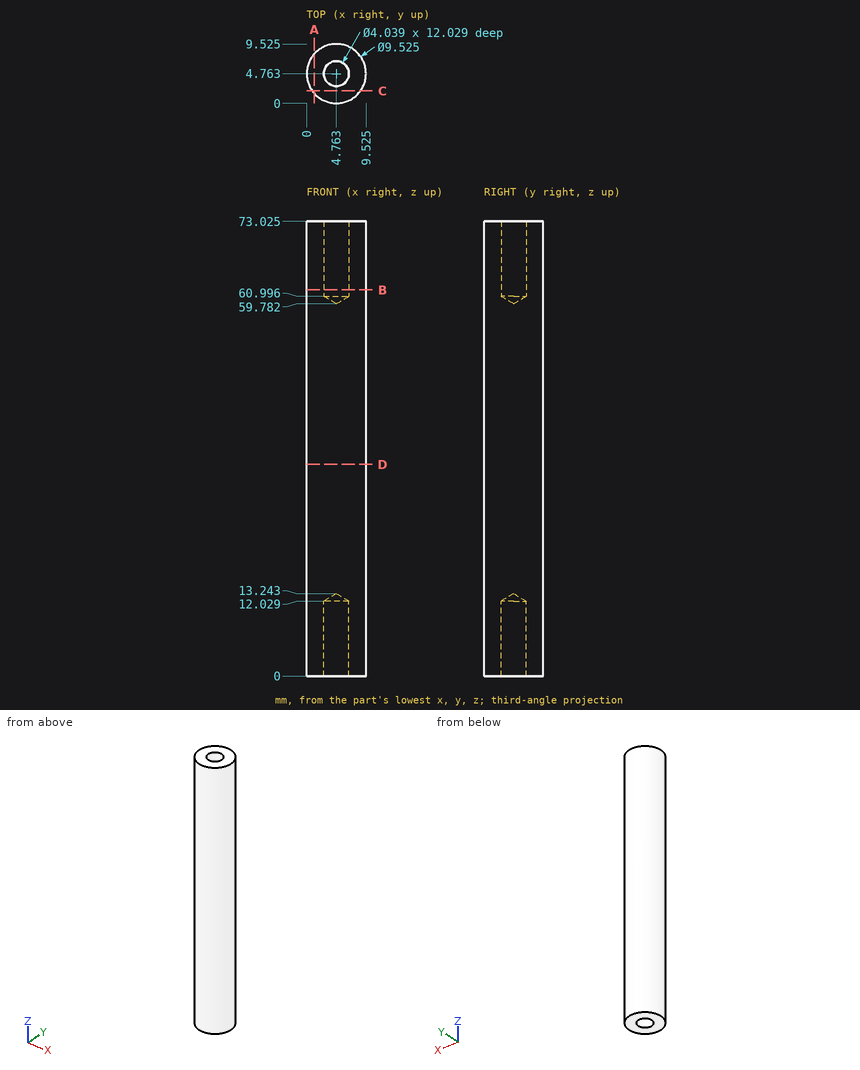
The drawing under review shows one solid part. Ordinate dimensions are in mm from its lowest x, y, z. Round coordinates to 2 decimals unless told otherwise and drop trailing zeros. Loops run counter-clockwise (first coordinate to the right, second up) from the corner with the lowest first, then second, coordinate; pieces in that order, holes last. Notation, with made-up numbers: (74.25, 8) - (98.25, 8) arc R18 ccw to (98.25, 32) - close; hole circle Ø10 at (16, 14). An arc over 180 degrees is marked (long way). Use a Markdown table: item, result. Add a question column.
Q1. Insertion check: pin 1 Ø2 at (x, y) = (5.5, 6.5) entering from -Z; pin 2 Ø1 at (x, z) = (8, 40) entering from -Y (1 decimal). Each pin has a flat end and moves straight along its axis. Give the tip position at first contact, or say it passes through.
Q2. Add section B-B (z = 62). State the section outline as (x, y) points (1 decimal).
Q3. Add section D-D (z = 34). State the section outline as (x, y) points (1 decimal).
Q4. Add section A-A (x = 1.25). State the section outline as (y, z) points (1 decimal), plus the area to 3 significant figures.
Q5. For probe 1 along X at (y, z) = (4.25, 69) (1 decimal); probe 2 along X at (y, z) = (7, 23) (1 decimal), list the stretches that pass through material, from the lowest coordinate up.
Q6. Add section C-C (y = 2). State the section outline as (x, z) points (1 decimal).
Worked answers:
| question | item | result |
|---|---|---|
| 1 | pin 1 | z = 0 |
| 1 | pin 2 | y = 0.9 |
| 2 | outline | circle Ø9.5 at (4.8, 4.8); hole circle Ø4 at (4.8, 4.8) |
| 3 | outline | circle Ø9.5 at (4.8, 4.8) |
| 4 | outline | (1.5, 0) - (8, 0) - (8, 73) - (1.5, 73) - close |
| 4 | area | 470 mm² |
| 5 | probe 1 | 0 to 2.8, 6.7 to 9.5 |
| 5 | probe 2 | 0.6 to 9 |
| 6 | outline | (0.9, 0) - (8.6, 0) - (8.6, 73) - (0.9, 73) - close |
